Verification items for the finished model (mm, model axes). A direction names the side the tool comes from. Give positions to 0.01 mm unless a question says otherwise; leave off trailing zeros. Loops run counter-clockwise (first coordinate to the right, second up) from the corner with the lowest first, then second, coordinate; pieces in that order, holes last. Notation, with made-up numbers: M 66,16.5 L 101,16.5 A19 ccw 101,35.5 Z; hole C -9,75 d11. An arc over 180 degrees is marked long. Use a Markdown table: item, result.
from build123d import *

# Parameters (mm, degrees)
F1_DEPTH = 25.4
F3_DEPTH = 25.4
F4_R     = 6.35
F5_DEPTH = 25.4
F7_DEPTH = 25.4


with BuildPart() as f1:
    # F0 (on Front) → F1 (new body)
    with BuildSketch(Plane.XZ):
        Polygon((0, 38.1), (0, 0), (69.85, 0), (69.85, 12.7), (25.4, 12.7), (25.4, 38.1), align=None)
    extrude(amount=F1_DEPTH)

    # F2 (on face) → F3 (cut)
    with BuildSketch(Plane.XY.offset(12.7)):
        with BuildLine():
            ThreePointArc((60.03999, 0), (66.500733, -2.88518), (69.85, -9.117986))
            Line((69.85, -9.117986), (69.85, 0))
            Line((69.85, 0), (60.03999, 0))
        make_face()
        with BuildLine():
            Line((69.85, -25.4), (69.85, -17.481705))
            ThreePointArc((69.85, -17.481705), (65.590949, -22.957802), (59.097659, -25.4))
            Line((59.097659, -25.4), (69.85, -25.4))
        make_face()
    extrude(amount=-F3_DEPTH, mode=Mode.SUBTRACT)

    # F4 (on face) → F5 (cut)
    with BuildSketch(Plane.XY.offset(38.1)):
        with Locations((12.7, -12.7)):
            Circle(F4_R)
    extrude(amount=-F5_DEPTH, mode=Mode.SUBTRACT)

    # F6 (on face) → F7 (cut)
    with BuildSketch(Plane.XY.offset(12.7)):
        with BuildLine():
            ThreePointArc((38.1, -19.05), (42.590128, -17.190128), (44.45, -12.7))
            ThreePointArc((44.45, -12.7), (42.590128, -8.209872), (38.1, -6.35))
            ThreePointArc((38.1, -6.35), (31.75, -12.7), (38.1, -19.05))
        make_face()
        with BuildLine():
            ThreePointArc((50.8, -6.35), (46.309872, -8.209872), (44.45, -12.7))
            ThreePointArc((44.45, -12.7), (46.309872, -17.190128), (50.8, -19.05))
            ThreePointArc((50.8, -19.05), (55.290128, -17.190128), (57.15, -12.7))
            ThreePointArc((57.15, -12.7), (55.290128, -8.209872), (50.8, -6.35))
        make_face()
        with BuildLine():
            ThreePointArc((50.8, -19.05), (46.309872, -17.190128), (44.45, -12.7))
            ThreePointArc((44.45, -12.7), (42.590128, -17.190128), (38.1, -19.05))
            Line((38.1, -19.05), (50.8, -19.05))
        make_face()
        with BuildLine():
            ThreePointArc((38.1, -6.35), (42.590128, -8.209872), (44.45, -12.7))
            ThreePointArc((44.45, -12.7), (46.309872, -8.209872), (50.8, -6.35))
            Line((50.8, -6.35), (38.1, -6.35))
        make_face()
    extrude(amount=-F7_DEPTH, mode=Mode.SUBTRACT)


solid = f1.part
(1) Gauge pin test, flat ends, axial feed: P1, Ø5, axis at y = -2.5, z = 27, coming from the +X side; P2, Ø5, axis at x = 28.5, z = 21, coming from the -Y side. Record the tip position at first contact, or that the pin passes through.
Results below:
| item | result |
|---|---|
| P1 | x = 25.4 |
| P2 | through |
(2) Draft check along Y on faces 1 (the flat face through (44, -19.05, 6)), 2 (the flat face through (0, -13, 19)), 3 (the cylindrical face through (65.67, -22.9, 6.44)). Enter one of: +Y half, -Y half, draft (parallel to the pull), parting line (faces both ways), or undercut.
Results below:
| item | result |
|---|---|
| face 1 | undercut |
| face 2 | draft |
| face 3 | -Y half |
(3) Set-up check for faces 4 (the flat face through (48, -21, 12.7)), 5 (the cylindrical face through (31.75, -12.56, 6.44)), 6 (the flat face through (13, -13, 12.7)): record each of +Z, -Z, +X, -X, +Y, -Y from which the full face is reachable in a straight line by a thin tool's end or side.
Results below:
| item | result |
|---|---|
| face 4 | +Z, +X, +Y, -Y |
| face 5 | +Z, -Z |
| face 6 | +Z |
(4) Cross-section at A-A on x = 42. Record the cut outline in (y, z), then the cut area to 3 significant figures.
Results below:
| item | result |
|---|---|
| outline | M -25.4,0 L -19.05,0 L -19.05,12.7 L -25.4,12.7 Z; M -6.35,0 L 0,0 L 0,12.7 L -6.35,12.7 Z |
| area | 161 mm^2 |
(5) Cross-section at B-B on z = 10. Record the cut outline in (x, y), then the cut area to 3 significant figures.
Results below:
| item | result |
|---|---|
| outline | M 0,-25.4 L 59.1,-25.4 A12.77 ccw 69.85,-17.48 L 69.85,-9.12 A10.95 ccw 60.04,0 L 0,0 Z; hole M 38.1,-19.05 L 50.8,-19.05 A6.35 ccw 50.8,-6.35 L 38.1,-6.35 A6.35 ccw Z |
| area | 1,440 mm^2 |
(6) Cross-section at D-D on x = 12.7. Record the cut outline in (y, z), then the cut area to 3 significant figures.
Results below:
| item | result |
|---|---|
| outline | M -25.4,0 L 0,0 L 0,38.1 L -6.35,38.1 L -6.35,12.7 L -19.05,12.7 L -19.05,38.1 L -25.4,38.1 Z |
| area | 645 mm^2 |
(7) Cross-section at C-C on y = -14.75. Record the cut outline in (x, z).
Results below:
| item | result |
|---|---|
| outline | M 0,0 L 32.09,0 L 32.09,12.7 L 25.4,12.7 L 25.4,38.1 L 18.71,38.1 L 18.71,12.7 L 6.69,12.7 L 6.69,38.1 L 0,38.1 Z; M 56.81,0 L 69.85,0 L 69.85,12.7 L 56.81,12.7 Z |
(8) Material ranges on line 1 (Y direction, x = 12.7, z = 30); line 2 (X direction, y = -13, z = 23); line 3 (Z direction, x = 36, y = -20.75), recorded low to high.
Results below:
| item | result |
|---|---|
| line 1 | -25.4 to -19.05, -6.35 to 0 |
| line 2 | 0 to 6.36, 19.04 to 25.4 |
| line 3 | 0 to 12.7 |
